```python
from build123d import *

# Parameters (mm, degrees)
SKETCH1_W           = 20
SKETCH1_H           = 240
BOSS_EXTRUDE1_DEPTH = 20
CUT_EXTRUDE1_DEPTH  = 20
SKETCH3_W           = 18
SKETCH3_H           = 18
CUT_EXTRUDE2_DEPTH  = 290


with BuildPart() as part:
    # Sketch1 → Boss-Extrude1 (new body)
    with BuildSketch(Plane.XY):
        with Locations((-51.462686567, -1.835820896)):
            Rectangle(SKETCH1_W, SKETCH1_H)
    extrude(amount=-BOSS_EXTRUDE1_DEPTH)

    # Sketch2 → Cut-Extrude1 (cut)
    with BuildSketch(Plane.ZY.offset(61.462686567)):
        Polygon((-20, 118.164179104), (0, 113.693649447), (0, 118.164179104), align=None)
    extrude(amount=-CUT_EXTRUDE1_DEPTH, mode=Mode.SUBTRACT)

    # Sketch3 → Cut-Extrude2 (cut)
    with BuildSketch(Plane.XZ.offset(121.835820896)):
        with Locations((-50.462686567, -9)):
            Rectangle(SKETCH3_W, SKETCH3_H)
    extrude(amount=-CUT_EXTRUDE2_DEPTH, mode=Mode.SUBTRACT)


solid = part.part
```
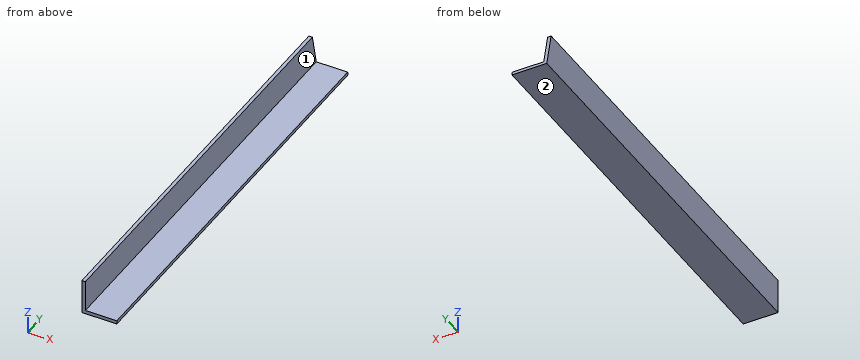
Can you work these out from the model? Positions are in its coordinate system, mm. Face numbers are marked on the shaded views. A direction names the side the tool comes from. Give positions to 0.01 mm unless a question says otherwise; leave off trailing zeros. Order: outer loops, then holes, each group sorted by start corner. A loop starts at its lowest first (then second) coordinate and runs counter-clockwise, first axis right, second up. Notation, with made-up numbers: M 18.25,-30.75 L 47.25,-30.75 A17 ccw 47.25,-19.75 Z; hole C 56,61.5 d1. An arc over 180 degrees is marked long. Write item = value, one per line. Start each with the question number.
Q1. Will these pins go through, and if not, where does the flat tip stop? pin 1 Ø9 at (x, y) = (-51.5, -31) entering from +Z; pin 2 Ø2 at (y, z) = (64.5, -13) entering from +X.
Q2. For the marked faces 1 and 2, which set-ups out of +Z, -Z, +X, -X, +Y, -Y let a thin tool reach every point of the face, with its end or its side?
Q3. Suppose I cut it at A-A (y = 98.5). Write out the boundary of the cut face in (x, z).
Q4. Suppose I cut it at C-C (z = -5.75). Write out the boundary of the cut face in (x, y), plus the area to 3 significant figures.
Q5. Suppose I cut it at B-B (x = -47.25). Write out the boundary of the cut face in (y, z), plus the area to 3 significant figures.
Q6. I need wall thicknesses on probe 1 along X at (y, z) = (54.5, -5.5); probe 2 along Z at (x, y) = (-56.5, 87). Which ranges of each line are inside material? Lowest first, please. Write a range as [from, to].
Check result:
q1.pin_1 = -18
q1.pin_2 = -59.46
q2.face_1 = +Z, +X, +Y, -Y
q2.face_2 = -Z, +X, -X, +Y, -Y
q3.outline = M -61.46,-20 L -41.46,-20 L -41.46,-18 L -59.46,-18 L -59.46,0 L -61.46,0 Z
q4.outline = M -61.46,-121.84 L -59.46,-121.84 L -59.46,114.98 L -61.46,114.98 Z
q4.area = 474 mm2
q5.outline = M -121.84,-20 L 118.16,-20 L 117.72,-18 L -121.84,-18 Z
q5.area = 480 mm2
q6.probe_1 = [-61.46, -59.46]
q6.probe_2 = [-20, -18]
